For this review, take the finished solid that the model builds, in its own axes (mm). A direction names the side the tool comes from. Coordinates: 2 decimals unless noted, no trailing zeros. One line per question, with ' | ' between items.
from build123d import *

# Parameters (mm, degrees)
SKETCH1_W             = 160
SKETCH1_H             = 30
BOSS_EXTRUDE1_DEPTH   = 0.6
SKETCH2_W             = 20
SKETCH2_H             = 20
SKETCH2_W_2           = 10
SKETCH2_H_2           = 10
SKETCH2_W_3           = 8
SKETCH2_H_3           = 8
SKETCH2_W_4           = 5
SKETCH2_H_4           = 5
SKETCH2_H_5           = 7
SKETCH2_H_6           = 12
SKETCH2_H_7           = 15
CUT_EXTRUDE1_DEPTH    = 0.6
CUT_EXTRUDE3_DEPTH    = 0.6
CUT_EXTRUDE4_DEPTH    = 0.6
CUT_EXTRUDE5_DEPTH    = 0.6
SKETCH7_W             = 9.123147958
SKETCH7_H             = 30
CUT_EXTRUDE6_DEPTH    = 0.6
BOSS_EXTRUDE2_DEPTH   = 0.6
BOSS_EXTRUDE2_2_DEPTH = 0.6
BOSS_EXTRUDE2_3_DEPTH = 0.6
BOSS_EXTRUDE2_4_DEPTH = 0.6
BOSS_EXTRUDE2_5_DEPTH = 0.6
BOSS_EXTRUDE2_6_DEPTH = 0.6
BOSS_EXTRUDE2_7_DEPTH = 0.6
BOSS_EXTRUDE2_8_DEPTH = 0.6
BOSS_EXTRUDE2_9_DEPTH = 0.6
FILLET1_R             = 3
SKETCH9_W             = 144.876852042
SKETCH9_H             = 1.5
BOSS_EXTRUDE3_DEPTH   = 0.6
CHAMFER1_SIZE         = 0.6


with BuildPart() as part:
    # Sketch1 → Boss-Extrude1 (new body)
    with BuildSketch(Plane(origin=(0, 0, 0), x_dir=(1, 0, 0), z_dir=(0, 1, 0))):
        Rectangle(SKETCH1_W, SKETCH1_H)
    extrude(amount=BOSS_EXTRUDE1_DEPTH)

    # Sketch2 → Cut-Extrude1 (cut)
    with BuildSketch(Plane(origin=(0, 0.6, 0), x_dir=(1, 0, 0), z_dir=(0, 1, 0))):
        with Locations((-65, 0)):
            Rectangle(SKETCH2_W, SKETCH2_H)
        with BuildLine():
            Line((-5, 12), (-7, 12))
            Line((-7, 12), (-7, 4))
            Line((-7, 4), (-5, 4))
            ThreePointArc((-5, 4), (-1, 8), (-5, 12))
        make_face()
        with Locations((-46, 7)):
            Rectangle(SKETCH2_W_2, SKETCH2_H_2)
        with Locations((-34, 6.702147352)):
            Rectangle(SKETCH2_W_3, SKETCH2_H_3)
        with Locations((-24.5, 7.5)):
            Rectangle(SKETCH2_W_4, SKETCH2_H_4)
        with Locations((-48.5, -6.5)):
            Rectangle(SKETCH2_W_4, SKETCH2_H_5)
        with BuildLine():
            Line((-15, 12), (-18, 12))
            Line((-18, 12), (-18, 2))
            Line((-18, 2), (-15, 2))
            ThreePointArc((-15, 2), (-10, 7), (-15, 12))
        make_face()
        with Locations((-40.5, -6.5)):
            Rectangle(SKETCH2_W_4, SKETCH2_H_3)
        with Locations((-32.5, -6)):
            Rectangle(SKETCH2_W_4, SKETCH2_H_6)
        with Locations((-24.5, -4.5)):
            Rectangle(SKETCH2_W_4, SKETCH2_H_7)
        with BuildLine():
            Line((3.5, 12), (2, 12))
            Line((2, 12), (2, 7))
            Line((2, 7), (3.5, 7))
            ThreePointArc((3.5, 7), (6, 9.5), (3.5, 12))
        make_face()
        with BuildLine():
            ThreePointArc((6.07040459, -2.329353078), (4.557646776, -6.329353078), (6.07040459, -10.329353078))
            add(Edge.make_bspline(
                [(6.07040459, -10.329353078), (-0.928342944, -10.345027892), (-3.92959541, -6.329353078)],
                knots=[0, 0, 0, 1, 1, 1], degree=2))
            add(Edge.make_bspline(
                [(6.07040459, -2.329353078), (-0.928342944, -2.313678264), (-3.92959541, -6.329353078)],
                knots=[0, 0, 0, 1, 1, 1], degree=2))
        make_face()
        with BuildLine():
            ThreePointArc((-5.087434715, -3.386719861), (-5.990420234, -6.386719861), (-5.087434715, -9.386719861))
            add(Edge.make_bspline(
                [(-5.087434715, -9.386719861), (-8.816275614, -9.455842755), (-12.087434715, -6.386719861)],
                knots=[0, 0, 0, 1, 1, 1], degree=2))
            add(Edge.make_bspline(
                [(-5.087434715, -3.386719861), (-8.816275614, -3.317596967), (-12.087434715, -6.386719861)],
                knots=[0, 0, 0, 1, 1, 1], degree=2))
        make_face()
        with BuildLine():
            ThreePointArc((-13.885876864, -4.386719861), (-14.307566838, -6.386719861), (-13.885876864, -8.386719861))
            add(Edge.make_bspline(
                [(-13.885876864, -8.386719861), (-17.299200456, -8.394557268), (-18.885876864, -6.386719861)],
                knots=[0, 0, 0, 1, 1, 1], degree=2))
            add(Edge.make_bspline(
                [(-13.885876864, -4.386719861), (-17.299200456, -4.378882454), (-18.885876864, -6.386719861)],
                knots=[0, 0, 0, 1, 1, 1], degree=2))
        make_face()
    extrude(amount=-CUT_EXTRUDE1_DEPTH, mode=Mode.SUBTRACT)

    # Sketch3 → Cut-Extrude3 (cut)
    with BuildSketch(Plane(origin=(0, 0.6, 0), x_dir=(1, 0, 0), z_dir=(0, 1, 0))):
        Polygon((10.717645067, 12), (10.717645067, -12), (15.717645067, -9.113248654), (15.717645067, 9.113248654), align=None)
        Polygon((19.717645067, 10), (19.717645067, -10), (24.717645067, -7.113248654), (24.717645067, 7.113248654), align=None)
        Polygon((28.717645067, 6), (28.717645067, -6), (33.717645067, -3.113248654), (33.717645067, 3.113248654), align=None)
    extrude(amount=-CUT_EXTRUDE3_DEPTH, mode=Mode.SUBTRACT)

    # Sketch5 → Cut-Extrude4 (cut)
    with BuildSketch(Plane(origin=(0, 0.6, 0), x_dir=(1, 0, 0), z_dir=(0, 1, 0))):
        Polygon((37.717645067, 10), (37.717645067, 1.5), (40.315721279, 0), (37.717645067, -1.5), (37.717645067, -10), (47.717645067, -4.226497308), (47.717645067, 4.226497308), align=None)
        Polygon((51.717645067, 6), (51.717645067, 1), (53.449695875, 0), (51.717645067, -1), (51.717645067, -6), (57.717645067, -2.535898385), (57.717645067, 2.535898385), align=None)
    extrude(amount=-CUT_EXTRUDE4_DEPTH, mode=Mode.SUBTRACT)

    # Sketch6 → Cut-Extrude5 (cut)
    with BuildSketch(Plane(origin=(0, 0.6, 0), x_dir=(1, 0, 0), z_dir=(0, 1, 0))):
        Polygon((63.758994289, 9.519130037), (61.258994289, 5.189003018), (66.258994289, 5.189003018), align=None)
        Polygon((63.484953651, -0.639697818), (59.484953651, -7.567901048), (67.484953651, -7.567901048), align=None)
    extrude(amount=-CUT_EXTRUDE5_DEPTH, mode=Mode.SUBTRACT)

    # Sketch7 → Cut-Extrude6 (cut)
    with BuildSketch(Plane(origin=(0, 0.6, 0), x_dir=(1, 0, 0), z_dir=(0, 1, 0))):
        with Locations((75.438426021, 0)):
            Rectangle(SKETCH7_W, SKETCH7_H)
    extrude(amount=-CUT_EXTRUDE6_DEPTH, mode=Mode.SUBTRACT)

    # Fillet1
    fillet1_edges = [part.edges().sort_by_distance(p)[0] for p in [
        (70.876852042, 0.3, 15),
        (70.876852042, 0.3, -15),
        (-80, 0.3, 15),
        (-80, 0.3, -15),
    ]]
    fillet(fillet1_edges, radius=FILLET1_R)



with BuildPart() as body_2:
    # Sketch8 → Boss-Extrude2 (new body)
    with BuildSketch(Plane(origin=(0, 0.6, 0), x_dir=(1, 0, 0), z_dir=(0, 1, 0))):
        Polygon((-75.472294668, 15), (-73.652443497, 20), (-67.292145839, 20), (-65.472294668, 15), align=None)
    extrude(amount=-BOSS_EXTRUDE2_DEPTH)


with BuildPart() as body_3:
    # Sketch8 → Boss-Extrude2 2 (new body)
    with BuildSketch(Plane(origin=(0, 0.6, 0), x_dir=(1, 0, 0), z_dir=(0, 1, 0))):
        Polygon((-59.112294668, 15), (-57.292443497, 20), (-50.932145839, 20), (-49.112294668, 15), align=None)
    extrude(amount=-BOSS_EXTRUDE2_2_DEPTH)


with BuildPart() as body_4:
    # Sketch8 → Boss-Extrude2 3 (new body)
    with BuildSketch(Plane(origin=(0, 0.6, 0), x_dir=(1, 0, 0), z_dir=(0, 1, 0))):
        Polygon((-42.752294668, 15), (-40.932443497, 20), (-34.572145839, 20), (-32.752294668, 15), align=None)
    extrude(amount=-BOSS_EXTRUDE2_3_DEPTH)


with BuildPart() as body_5:
    # Sketch8 → Boss-Extrude2 4 (new body)
    with BuildSketch(Plane(origin=(0, 0.6, 0), x_dir=(1, 0, 0), z_dir=(0, 1, 0))):
        Polygon((-26.392294668, 15), (-24.572443497, 20), (-18.212145839, 20), (-16.392294668, 15), align=None)
    extrude(amount=-BOSS_EXTRUDE2_4_DEPTH)


with BuildPart() as body_6:
    # Sketch8 → Boss-Extrude2 5 (new body)
    with BuildSketch(Plane(origin=(0, 0.6, 0), x_dir=(1, 0, 0), z_dir=(0, 1, 0))):
        Polygon((-10.032294668, 15), (-8.212443497, 20), (-1.852145839, 20), (-0.032294668, 15), align=None)
    extrude(amount=-BOSS_EXTRUDE2_5_DEPTH)


with BuildPart() as body_7:
    # Sketch8 → Boss-Extrude2 6 (new body)
    with BuildSketch(Plane(origin=(0, 0.6, 0), x_dir=(1, 0, 0), z_dir=(0, 1, 0))):
        Polygon((6.327705332, 15), (8.147556503, 20), (14.507854161, 20), (16.327705332, 15), align=None)
    extrude(amount=-BOSS_EXTRUDE2_6_DEPTH)


with BuildPart() as body_8:
    # Sketch8 → Boss-Extrude2 7 (new body)
    with BuildSketch(Plane(origin=(0, 0.6, 0), x_dir=(1, 0, 0), z_dir=(0, 1, 0))):
        Polygon((22.687705332, 15), (24.507556503, 20), (30.867854161, 20), (32.687705332, 15), align=None)
    extrude(amount=-BOSS_EXTRUDE2_7_DEPTH)


with BuildPart() as body_9:
    # Sketch8 → Boss-Extrude2 8 (new body)
    with BuildSketch(Plane(origin=(0, 0.6, 0), x_dir=(1, 0, 0), z_dir=(0, 1, 0))):
        Polygon((39.047705332, 15), (40.867556503, 20), (47.227854161, 20), (49.047705332, 15), align=None)
    extrude(amount=-BOSS_EXTRUDE2_8_DEPTH)


with BuildPart() as body_10:
    # Sketch8 → Boss-Extrude2 9 (new body)
    with BuildSketch(Plane(origin=(0, 0.6, 0), x_dir=(1, 0, 0), z_dir=(0, 1, 0))):
        Polygon((55.407705332, 15), (57.227556503, 20), (63.587854161, 20), (65.407705332, 15), align=None)
    extrude(amount=-BOSS_EXTRUDE2_9_DEPTH)


with BuildPart() as part_1:
    add(part.part)

    add(body_2.part)  # Boss-Extrude3 merges body 2

    add(body_3.part)  # Boss-Extrude3 merges body 3

    add(body_4.part)  # Boss-Extrude3 merges body 4

    add(body_5.part)  # Boss-Extrude3 merges body 5

    add(body_6.part)  # Boss-Extrude3 merges body 6

    add(body_7.part)  # Boss-Extrude3 merges body 7

    add(body_8.part)  # Boss-Extrude3 merges body 8

    add(body_9.part)  # Boss-Extrude3 merges body 9

    add(body_10.part)  # Boss-Extrude3 merges body 10
    # Sketch9 → Boss-Extrude3 (add)
    with BuildSketch(Plane(origin=(0, 0.6, 0), x_dir=(1, 0, 0), z_dir=(0, 1, 0))):
        with Locations((-4.561573979, 14.25)):
            Rectangle(SKETCH9_W, SKETCH9_H)
        with Locations((-4.561573979, -14.25)):
            Rectangle(SKETCH9_W, SKETCH9_H)
    extrude(amount=BOSS_EXTRUDE3_DEPTH)

    # Chamfer1
    chamfer1_edges = [part_1.edges().sort_by_distance(p)[0] for p in [
        (67.876852042, 1.2, 14.25),
        (67.876852042, 1.2, -14.25),
        (-77, 1.2, 14.25),
        (-77, 1.2, -14.25),
    ]]
    chamfer(chamfer1_edges, length=CHAMFER1_SIZE - 0.0001)  # a hair under: the kernel refuses the full size


solid = part_1.part
1) We need section A-A on y = 0.3. State how many separate pieces and enclosed holes the cut face has, then the cut area to 3 significant figures.
Responses:
separate pieces: 1 | enclosed holes: 21 | area: 3,410 mm^2
2) Insertion check: pin 1 Ø5 at (x, z) = (-4, -2.5) entering from +Y. The pin has a flat end and moves straight along its axis. Give the tip position at first contact, or say it passes through.
Responses:
pin 1: y = 0.6
3) Machinability: for faces 5 (the cylindrical face through (69.975, 0.296, -14.145)), 6 (the cylindrical face through (6, 0.3, -9.4)), 7 (the flat face through (28, 0.6, -18)), which of the approach directions +Z, -Z, +X, -X, +Y, -Y give a long, thin tool a straight path to every point of the face, cutting with its end or side? Answer none if there is none.
Responses:
face 5: -Z, +X, +Y, -Y | face 6: +Y, -Y | face 7: -Z, +X, -X, +Y
4) The part is to be moulded in two halves that separate along Z. For faces 1 (the cylindrical face through (69.975, 0.296, 14.145)), 2 (the flat face through (13.25, 0.3, -10.54)), 3 (the flat face through (-71, 0.6, -18)), 4 (the cylindrical face through (-1, 0.3, -7.9)), say which applies: +Z half, -Z half, draft (parallel to the pull), parting line (faces both ways), or undercut.
Responses:
face 1: +Z half | face 2: undercut | face 3: draft | face 4: undercut
5) To check wall thickness, follow line 1 along Z through (x, y) = (-24.5, 1); line 2 along Z through (x, y) = (-68, 0.5); line 3 along Z through (x, y) = (35, 0.35). State the ranges of each line that lie inside material, in increasing order. Write a range as [from, to].
Responses:
line 1: [-15, -13.5], [13.5, 15] | line 2: [-20, -10], [10, 15] | line 3: [-15, 15]
